Can you work these out from the model? Positions are in its coordinate system, mm. A direction names the side the tool comes from. Give positions to 0.01 mm unless a question says otherwise; leave off trailing zeros. Order: outer loops, then holes, each group sorted by start corner. A loop starts at its lowest first (then second) coordinate and runs counter-clockwise, first axis right, second up.
Autodesk Inventor part; units mm, degrees
ref_plane "Work Plane1" through (1.525, 0, 0) normal (0, 0, 1) x (1, 0, 0)
ref_plane "YZ Plane" through (0, 0, 0) normal (1, 0, 0) x (0, 1, 0)
ref_plane "XZ Plane" through (0, 0, 0) normal (0, 1, 0) x (-1, 0, 0)
sketch "Sketch1" plane through (0, 0, 0) normal (0, 0, 1) x (1, 0, 0)
  line L0 (0, 3.5) -> (42, 3.5)
  line L1 (42, 3.5) -> (42, 0)
  line L2 (42, 0) -> (0, 0)
  line L3 (-8.4, 0) -> (50.4, 0)
  line L4 (0, -0.7) -> (0, 4.2)
  line L5 (0, 3.5) -> (0, 0)
  dimension "d2" = 7
  dimension "d59" = 42
revolve "Body" add sketch "Sketch1" angle 360 about axis through (42, 0, 0) along (-1, 0, 0)
sketch "Sketch2" plane through (0, 0, 0) normal (-1, 0, 0) x (0, 0, 1)
  line L0 (0, 6.3509) -> (5.5, 3.1754)
  line L1 (5.5, 3.1754) -> (5.5, -3.1754)
  line L2 (5.5, -3.1754) -> (0, -6.3509)
  line L3 (0, -6.3509) -> (-5.5, -3.1754)
  line L4 (-5.5, -3.1754) -> (-5.5, 3.1754)
  line L5 (-5.5, 3.1754) -> (0, 6.3509)
  line L6 (-7.7, 0) -> (7.7, 0)
  line L7 (0, 8.8912) -> (0, -8.8912)
  point P0 (0, 0)
  point P1 (0, 0)
  dimension "d11" = 11
extrude "Head" add sketch "Sketch2" along normal blind 4.5
sketch "Sketch4" plane through (0, 0, 0) normal (0, 0, 1) x (1, 0, 0)
  line L0 (-3.8649, 6.6) -> (-4.5, 5.5)
  line L1 (-1.1, 0) -> (-0.234, 0)
  line L2 (-5.3532, 0) -> (0.6192, 0)
  line L3 (-4.5, 6.6) -> (-3.8649, 6.6)
  line L4 (-4.5, 5.5) -> (-4.5, 6.6)
  line L5 (0, 7.92) -> (0, -1.32)
  dimension "d65" = 11
  dimension "d67" = 30
  dimension "d68" = 13.2
  dimension "d69" = 4.5
revolve "Chamfer1" cut sketch "Sketch4" angle 360 about axis through (-1.1, 0, 0) along (1, 0, 0)
thread "Thread"
chamfer "Chamfer2" distance 0.6135 distance2 0.6136 1 edges at (42, -3.5, 0) measured on face at (42, -1.0838, 0.9601)
fillet "Fillet2" radius 0.3 1 edges at (0, -3.5, 0)
ref_plane "Work Plane1" through (1.525, 0, 0) normal (0, 0, 1) x (1, 0, 0)
equation "\"d2\" = GD"
equation "\"d59\" = NLG"
equation "\"d11\" = SW"
equation "\"d3\" = KOH"
equation "\"d71\" = RR"
equation "\"d15\" = GEL"
equation "\"d6\" = -0.5 * SPD + 0.5 * GD"
equation "\"d65\" = SW"
equation "\"d67\" = ANG1"
equation "\"d68\" = 1.2 * SW"
equation "\"d69\" = KOH"
equation "\"NLG\" = 42"
equation "\"GD\" = NND"
equation "\"BDM\" = NND"
equation "\"KOH\" = 4.5"
equation "\"GEL\" = 13"
equation "\"SW\" = 11"
equation "\"SW0\" = 11"
equation "\"SPD\" = NND - 1.2269 * PTC"
equation "\"SD2\" = NND"
equation "\"SD\" = 0"
equation "\"ANG1\" = 30deg"
equation "\"GAL\" = 0.61345 * PTC"
equation "\"GUL\" = 0.61345 * PTC"
equation "\"RR\" = 0.3"
equation "\"RR1\" = 0.1"
equation "\"GD1\" = THREADDIA - 1.2269 * PTC"
equation "\"THREADDIA\" = 7"
equation "\"TOA\" = 30deg"
equation "\"FAWI\" = 60deg"
equation "\"PTC\" = 1"
equation "\"NND\" = 7"
equation "\"E0\" = 1.155 * SW"
properties part number "CSN 02 1201 - M7 x 42" material "Steel, Mild"
1) If I drill on line 1 (X direction, y = 3, z = -4); line 2 (Y direction, x = 5.5, z = -0.25); line 3 (Z direction, x = 28.5, y = -2), over which ranges is the centre line in solid material (lowest first)?
2) Which directions (+Z, -Z, +X, -X, +Y, -Y) give clear straight access to the entire face, cutting with the end or side of a thin tool? Please do faces 1 (the face through (-4.5, 0, 0)), 2 (the face through (21.131, 3.233, -1.341)).
3) I'm going to push flat-ended pins straight in: pin 1 Ø2 at (x, z) = (15, 1.5) entering from -Y; pin 2 Ø6 at (x, y) = (18.5, 1.5) entering from +Z; pin 3 Ø3 at (x, y) = (33, -4) entering from +Z; pin 4 Ø6 at (y, z) = (5, 3) entering from +X. Where does each tip first touch, or does it pass through?
4) Suppose I cut it at A-A (x = 39). Please give me the cut outline in (y, z), and give its area (3 significant figures).
Results:
1. line 1: x = -4.5 to 0
1. line 2: y = -3.49 to 3.49
1. line 3: z = -2.87 to 2.87
2. face 1: +Z, -Z, -X, +Y, -Y
2. face 2: +X
3. pin 1: stops at y = -3.46
3. pin 2: stops at z = 3.5
3. pin 3: stops at z = 2.45
3. pin 4: stops at x = 42
4. outline: circle Ø7 at (0, 0)
4. area: 38.5 mm2
